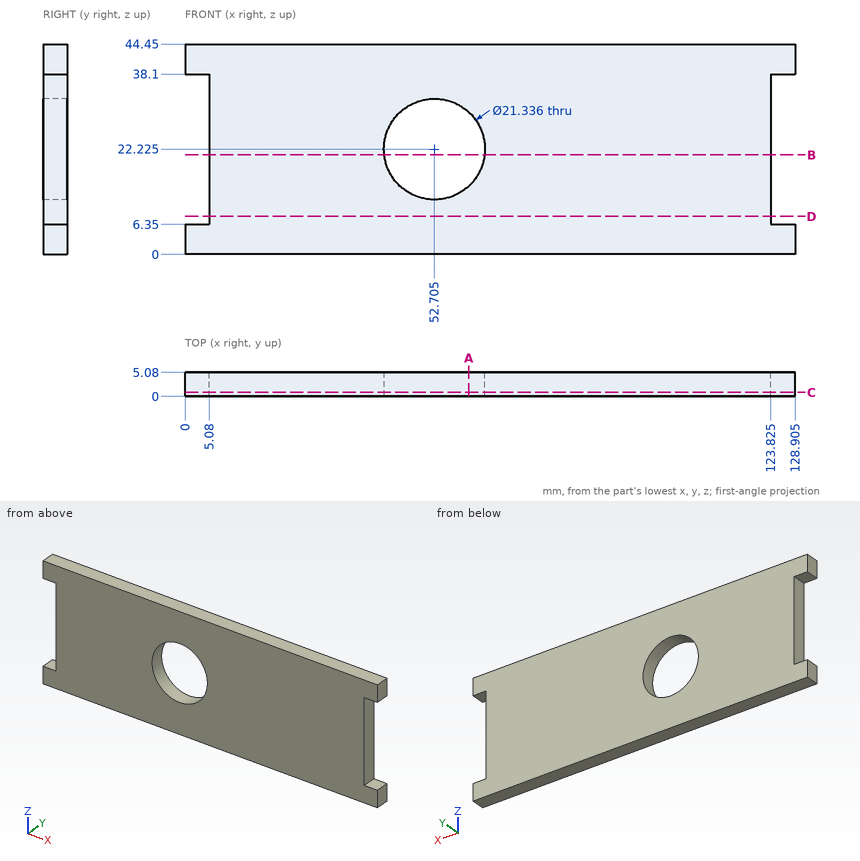
Verification items for this drawing (mm, ordinates from the low corner). Round coordinates to 2 decimals unless told otherwise and drop trailing zeros. Loops run counter-clockwise (first coordinate to the right, second up) from the corner with the lowest first, then second, coordinate; pieces in that order, holes last. Notation, with made-up numbers: (43, 74) - (96, 74) arc R3 ccw to (96, 79) - close; hole circle Ø8 at (-29.75, -25.75). An arc over 180 degrees is marked (long way). Answer as CSV lines item,"result". Start each with the question number.
Item 1: Scan lines: line 1 (Z direction, x = 51, y = 1.3); line 2 (X direction, y = 2.05, z = 19) (3 decimals); line 3 (X direction, y = 2.4, z = 11) (3 decimals). Record each from-to range of solid material in increasing order. Write a range as [from, to].
Item 2: Section check A-A (x = 60). Record the boundary of the cut face in (y, z).
Item 3: Depth check by flat-ended pin: P1, Ø3, axis at y = 3, z = 33.5, coming from the -X side. Enter the tip coordinate at first touch or a pass-through.
Item 4: Section check C-C (y = 0.85). Record the boundary of the cut face in (x, z) (3 decimals).
Item 5: Section check D-D (z = 8). Record the boundary of the cut face in (x, y) (3 decimals).
Item 6: Section check B-B (z = 21). Record the boundary of the cut face in (x, y) (3 decimals), and give its area (3 significant figures).
Report:
1,line 1,"z = [0, 11.69], [32.76, 44.45]"
1,line 2,"x = [5.08, 42.536], [62.874, 123.825]"
1,line 3,"x = [5.08, 123.825]"
2,outline,"(0, 0) - (5.08, 0) - (5.08, 14.44) - (0, 14.44) - close; (0, 30.01) - (5.08, 30.01) - (5.08, 44.45) - (0, 44.45) - close"
3,P1,"stops at x = 5.08"
4,outline,"(0, 0) - (128.905, 0) - (128.905, 6.35) - (123.825, 6.35) - (123.825, 38.1) - (128.905, 38.1) - (128.905, 44.45) - (0, 44.45) - (0, 38.1) - (5.08, 38.1) - (5.08, 6.35) - (0, 6.35) - close; hole circle Ø21.336 at (52.705, 22.225)"
5,outline,"(5.08, 0) - (123.825, 0) - (123.825, 5.08) - (5.08, 5.08) - close"
6,outline,"(5.08, 0) - (42.108, 0) - (42.108, 5.08) - (5.08, 5.08) - close; (63.302, 0) - (123.825, 0) - (123.825, 5.08) - (63.302, 5.08) - close"
6,area,"496 mm2"
